```python
from build123d import *

# Parameters (mm, degrees)
SKETCH1_R      = 20
EXTRUDE1_DEPTH = 25
EXTRUDE2_DEPTH = 38
EXTRUDE3_DEPTH = 38


with BuildPart() as part:
    # Sketch1 → Extrude1 (new body)
    with BuildSketch(Plane.XY):
        Circle(SKETCH1_R)
    extrude(amount=EXTRUDE1_DEPTH)

    # Sketch2 → Revolve1 (revolve)
    with BuildSketch(Plane(origin=(0, 0, 0), x_dir=(0, 0, -1), z_dir=(1, 0, 0))):
        with BuildLine():
            Line((-25, 0), (-35.80749354, 0))
            ThreePointArc((-35.80749354, 0), (-33.08089551, 11.446663385), (-25, 20))
            Line((-25, 20), (-25, 0))
        make_face()
    revolve(axis=Axis((0, 0, 25), (0, 0, 1)))

    # Sketch3 → Extrude2 (add)
    with BuildSketch(Plane(origin=(0, 0, 0), x_dir=(0, 0, -1), z_dir=(1, 0, 0))):
        with BuildLine():
            ThreePointArc((-17, -16), (-8.838692689, -0.914824388), (-6, 16))
            ThreePointArc((-6, 16), (-7, 16.414213562), (-8, 16))
            ThreePointArc((-8, 16), (-10.94657476, -0.304222576), (-18.7, -14.946434625))
            ThreePointArc((-18.7, -14.946434625), (-18.068200534, -15.82529884), (-17, -16))
        make_face()
    extrude(amount=EXTRUDE2_DEPTH)

    # Sketch4 → Extrude3 (add)
    with BuildSketch(Plane(origin=(0, 0, 0), x_dir=(0, 0, -1), z_dir=(1, 0, 0))):
        with BuildLine():
            ThreePointArc((-8, -16), (-7, -16.312065741), (-6, -16))
            ThreePointArc((-6, -16), (-8.838692689, 0.914824388), (-17, 16))
            ThreePointArc((-17, 16), (-18.068200534, 15.82529884), (-18.7, 14.946434625))
            ThreePointArc((-18.7, 14.946434625), (-10.94657476, 0.304222576), (-8, -16))
        make_face()
    extrude(amount=-EXTRUDE3_DEPTH)


solid = part.part
```
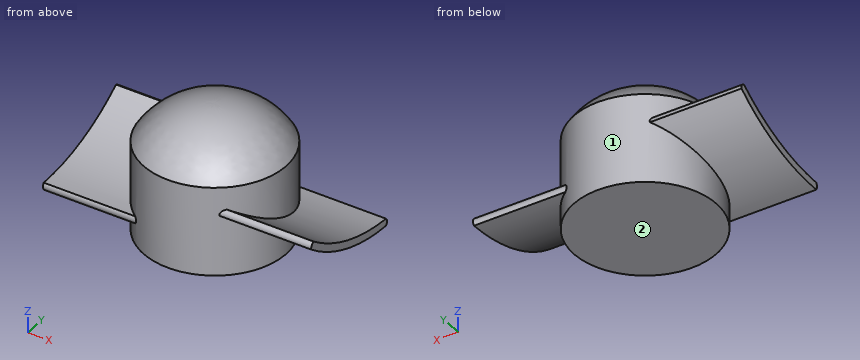
Here's how the part is built. I have some questions about the finished solid (model axes, mm). Face numbers are marked on the shaded views. A direction names the side the tool comes from. Give positions to 0.01 mm unless a question says otherwise; leave off trailing zeros. Order: outer loops, then holes, each group sorted by start corner. A loop starts at its lowest first (then second) coordinate and runs counter-clockwise, first axis right, second up. Notation, with made-up numbers: (16, -4.75) - (72, -4.75) arc R15 cw to (72, 12.25) - close; hole circle Ø10 at (82.25, 53). An arc over 180 degrees is marked (long way). Answer as a JSON object with one key per item and string values. Group by question number.
Item 1: Which directions (+Z, -Z, +X, -X, +Y, -Y) give clear straight access to the entire face, cutting with the end or side of a thin tool? Please do the marked faces 1 and 2.
Item 2: If we section it at A-A on z = 9.5: Please give me the cut outline in (x, y).
Item 3: Please list where these lines run through material, in increasing order: probe 1 along Y at (x, z) = (-14.5, 18.5); probe 2 along X at (y, z) = (16, 7.5); probe 3 along Z at (x, y) = (-24, 1).
Item 4: For P1, Ø10, axis at y = 14, z = 5.5, coming from the -X side; P2, Ø2, axis at y = -5.5, z = 4, coming from the +X side; P3, Ø12, axis at x = -9.5, z = 29.5, coming from the +Y side; P4, Ø6, axis at x = -9.5, y = -9, coming from the -Z side, each with a flat end and sliding along its axis, tell me the tip position at first contact or that it passes through.
Result set:
{
 "1": {"face 1": "none", "face 2": "-Z, +X, -X, +Y, -Y"},
 "2": {"outline": "(-38, -4.63) - (-19.46, -4.63) arc R20 ccw to (19.81, -2.73) - (38, -2.73) - (38, 4.63) - (19.46, 4.63) arc R20 ccw to (-19.81, 2.73) - (-38, 2.73) - close"},
 "3": {"probe 1": "-13.77 to 13.77, 14.68 to 15.41", "probe 2": "-12 to 38", "probe 3": "8.87 to 11.19"},
 "4": {"P1": "x = -17.86", "P2": "x = 19.49", "P3": "y = 19.22", "P4": "z = 0"}
}
